Autodesk Inventor part; units mm, degrees
ref_plane "작업 평면1" through (126.678, -21.6572, 32.6995) normal (0, 0.8660254, 0.5) x (1, 0, 0)
ref_plane "YZ Plane" through (0, 0, 0) normal (1, 0, 0) x (0, 1, 0)
ref_plane "XZ Plane" through (0, 0, 0) normal (0, 1, 0) x (-1, 0, 0)
ref_plane "작업 평면1" through (126.678, -21.6572, 32.6995) normal (0, 0.8660254, 0.5) x (1, 0, 0)
sketch "스케치1" plane through (126.678, -21.6572, 32.6995) normal (0, 0.8660254, 0.5) x (1, 0, 0)
  circle A0 centre (89.9, 9) radius 1.5
  circle A1 centre (-89.9, -1) radius 1.5
  circle A2 centre (-89.9, 9) radius 1.5
  circle A3 centre (89.9, -1) radius 1.5
  circle A4 centre (32.9, 9) radius 1.5
  circle A5 centre (-32.9, -1) radius 1.5
  circle A6 centre (-32.9, 9) radius 1.5
  circle A7 centre (32.9, -1) radius 1.5
  line L0 (95, -17) -> (95, 17)
  line L1 (8, 17) -> (95, 17)
  line L2 (8, 17) -> (8, 10)
  arc A8 (6, 8) -> (8, 10) centre (6, 10) ccw
  line L3 (6, 8) -> (-6, 8)
  arc A9 (-8, 10) -> (-6, 8) centre (-6, 10) ccw
  line L4 (-8, 10) -> (-8, 17)
  line L5 (-95, 17) -> (-8, 17)
  line L6 (-95, 17) -> (-95, -17)
  line L7 (95, -17) -> (-95, -17)
  line L8 (95, 13) -> (95, -20)
  line L9 (95, -20) -> (-95, -20)
  line L10 (-95, -20) -> (-95, 13)
  line L11 (-95, 13) -> (-84.8, 13)
  line L12 (-84.8, 13) -> (-84.8, -5)
  line L13 (-84.8, -5) -> (-95, -5)
  line L14 (-95, -5) -> (-95, 13)
  line L15 (-38, 13) -> (-27.8, 13)
  line L16 (-27.8, 13) -> (-27.8, -5)
  line L17 (-27.8, -5) -> (-38, -5)
  line L18 (-38, -5) -> (-38, 13)
  line L19 (27.8, 13) -> (38, 13)
  line L20 (38, 13) -> (38, -5)
  line L21 (38, -5) -> (27.8, -5)
  line L22 (27.8, -5) -> (27.8, 13)
  line L23 (95, 13) -> (84.8, 13)
  line L24 (84.8, 13) -> (84.8, -5)
  line L25 (84.8, -5) -> (95, -5)
  line L26 (95, -5) -> (95, 13)
  line L27 (-84.8, -5) -> (84.8, -5)
  line L28 (84.8, 13) -> (95, 13)
  line L29 (27.8, 13) -> (38, 13)
  line L30 (-95, 13) -> (-84.8, 13)
  line L31 (-38, 13) -> (-27.8, 13)
  point P0 (-126.678, 39.1472)
  dimension "d1" = 190
  dimension "d2" = 33
  dimension "d5" = 10.2
  dimension "d6" = 18
  dimension "d7" = 10.2
  dimension "d8" = 18
  dimension "d9" = 10.2
  dimension "d10" = 18
  dimension "d11" = 5.1
  dimension "d12" = 18
  dimension "d13" = 10.2
  dimension "d14" = 5.1
extrude "돌출1" add sketch "스케치1" along normal blind 2 contours L7 L6 L13 L27 L17 L21 L25 L0 | L8 L9 L10 L7 | L25 L24 L23 L0 | L6 L11 L12 L13 | L21 L22 L19 L20 | L18 L15 L16 L17
sketch "스케치2" plane through (126.678, -19.9251, 33.6995) normal (0, 0.8660254, 0.5) x (1, 0, 0)
  circle A0 centre (32.9, 9) radius 1.5
  circle A1 centre (32.9, -1) radius 1.5
  circle A2 centre (-89.9, 9) radius 1.5
  circle A3 centre (-89.9, -1) radius 1.5
  circle A4 centre (89.9, 9) radius 1.5
  circle A5 centre (89.9, -1) radius 1.5
  circle A6 centre (-32.9, 9) radius 1.5
  circle A7 centre (-32.9, -1) radius 1.5
  line L0 (-38, 13) -> (-38, -5)
  line L1 (-38, -5) -> (-84.8, -5)
  line L2 (-84.8, -5) -> (-84.8, 13)
  line L3 (-84.8, 13) -> (-95, 13)
  line L4 (-95, 13) -> (-95, -20)
  line L5 (-95, -20) -> (95, -20)
  line L6 (95, -20) -> (95, 13)
  line L7 (95, 13) -> (84.8, 13)
  line L8 (84.8, 13) -> (84.8, -5)
  line L9 (84.8, -5) -> (38, -5)
  line L10 (38, -5) -> (38, 13)
  line L11 (38, 13) -> (27.8, 13)
  line L12 (27.8, 13) -> (27.8, -5)
  line L13 (27.8, -5) -> (-27.8, -5)
  line L14 (-27.8, -5) -> (-27.8, 13)
  line L15 (-27.8, 13) -> (-38, 13)
  line L16 (-95, -20) -> (95, -20)
  line L17 (-86, -20) -> (-86, -12)
  line L18 (-86, -12) -> (-70, -12)
  line L19 (-70, -12) -> (-50, -12)
  line L20 (-50, -12) -> (-30, -12)
  line L21 (-30, -12) -> (-10, -12)
  line L22 (-10, -12) -> (10, -12)
  line L23 (10, -12) -> (30, -12)
  line L24 (30, -12) -> (50, -12)
  line L25 (50, -12) -> (70, -12)
  line L26 (70, -12) -> (86, -12)
  circle A8 centre (-86, -12) radius 1.5
  circle A9 centre (-70, -12) radius 1.5
  circle A10 centre (-50, -12) radius 1.5
  circle A11 centre (-30, -12) radius 1.5
  circle A12 centre (-10, -12) radius 1.5
  circle A13 centre (10, -12) radius 1.5
  circle A14 centre (30, -12) radius 1.5
  circle A15 centre (50, -12) radius 1.5
  circle A16 centre (70, -12) radius 1.5
  circle A17 centre (86, -12) radius 1.5
  point P0 (-126.678, 39.1472)
  dimension "d17" = 8
  dimension "d18" = 16
  dimension "d19" = 20
  dimension "d20" = 20
  dimension "d21" = 20
  dimension "d22" = 20
  dimension "d23" = 20
  dimension "d24" = 20
  dimension "d25" = 20
  dimension "d26" = 16
  dimension "d27" = 9
  dimension "d28" = 3
  dimension "d29" = 3
  dimension "d30" = 3
  dimension "d31" = 3
  dimension "d32" = 3
  dimension "d33" = 3
  dimension "d34" = 3
  dimension "d35" = 3
  dimension "d36" = 3
  dimension "d38" = 3
extrude "돌출2" cut sketch "스케치2" against normal blind 1 contours A8 L18 L17 | L17 L18 A8 | A9 L19 L18 | L18 L19 A9 | A10 L20 L19 | L19 L20 A10 | A11 L21 L20 | L20 L21 A11 | A12 L22 L21 | L21 L22 A12 | A13 L23 L22 | L22 L23 A13 | A14 L24 L23 | L23 L24 A14 | A15 L25 L24 | L24 L25 A15 | A16 L26 L25 | L25 L26 A16 | A17
properties part number "칼팁" material "철, 주조"
Verification items for the finished model (mm, model axes). Give positions to 0.01 mm unless a question says otherwise; leave off trailing zeros. Write each loop counter-clockwise with the first axis right and the second up, starting at its lowest first coordinate (ties: lowest second). Pieces come first, ordered by that corner, then holes. Notation, with made-up numbers: M -28,29 L 20,29 A17 cw 20,34 Z; hole C 41,11.5 d1. An arc over 180 degrees is marked long. One line per question, with ' | ' between items.
1) Section check B-B on x = 183. Enter the section's corners in (y, z).
Result:
outline: M -31.66,50.02 L -24.16,37.03 L -22.43,38.03 L -29.93,51.02 Z
2) Section check A-A on z = 29. Enter the section's corners in (x, y).
Result:
outline: M 31.68,-19.52 L 41.88,-19.52 L 41.88,-17.21 L 31.68,-17.21 Z; M 88.68,-19.52 L 98.88,-19.52 L 98.88,-17.21 L 88.68,-17.21 Z; M 154.48,-19.52 L 164.68,-19.52 L 164.68,-17.21 L 154.48,-17.21 Z; M 211.48,-19.52 L 221.68,-19.52 L 221.68,-17.21 L 211.48,-17.21 Z
3) Gauge pin test, flat ends, axial feed: pin 1 Ø10 at (y, z) = (-27.5, 41.5) entering from -X; pin 2 Ø5 at (x, z) = (96, 42.5) entering from +Y; pin 3 Ø6 at (x, y) = (184, -28.5) entering from +Z; pin 4 Ø3 at (x, z) = (131, 38.5) entering from -Y. Record the tip position at first contact, or that the pin passes through.
Result:
pin 1: stops at x = 31.68 | pin 2: stops at y = -23.56 | pin 3: stops at z = 51.02 | pin 4: stops at y = -25.87
4) Thickness scan on line 1 along Z through (x, y) = (203, -27.75); line 2 along Y through (x, z) = (116, 38); line 3 along Y through (x, z) = (48.5, 44). Record the ranges inside material, lowest first. Write a range as [from, to].
Result:
line 1: z = [43.25, 47.25] | line 2: y = [-24.72, -22.48] | line 3: y = [-28.18, -25.87]
5) Mould release check, pull along Z, two halves, no side actions. Record for faces 1 (the cylindrical face through (118.064, -26.64, 44.342)), 2 (the flat face through (154.478, -19, 30)), 3 (the flat face through (125.348, -26.958, 41.881)): released by +Z, released by -Z, zero draft, split by the parting line, or undercut.
Result:
face 1: undercut | face 2: zero draft | face 3: released by -Z
